Part model, mm, in its own coordinate system. Face numbers are marked on the shaded views. A direction names the side the tool comes from. Coordinates: 2 decimals unless noted, no trailing zeros. Order: outer loops, then holes, each group sorted by start corner. A loop starts at its lowest first (then second) coordinate and runs counter-clockwise, first axis right, second up.
1) Cut at C-C (y = -6.5). List the corners of the cut face in (x, z).
2) Cut at D-D (z = 24.5). List the corners of the cut face in (x, y) (3 decimals), and give its area (3 significant figures).
3) Pin check, flat tips, straight feed: pin 1 Ø6 at (y, z) = (-5.5, 20) entering from -X; pin 2 Ø1 at (y, z) = (1, 9) entering from -X; pin 3 Ø1 at (x, z) = (-1, 26) entering from +Y. Stop position of each tip, or through.
4) Wall check: L1, parallel to Y at x = 0, z = 7.5 (3 decimals); L2, parallel to Y at x = -2.75, z = 11.5; L3, parallel to X at y = -4.25, z = 8.5. Give the ranges that are in metal, low to high.
5) Cut at A-A (x = 0). List the corners of the cut face in (y, z) (3 decimals).
6) Cut at B-B (z = 15). List the corners of the cut face in (x, y) (3 decimals).
7) Mould opens along Y. For the marked faces 3, 4 and 5 say: +Y half, -Y half, draft (parallel to the pull), parting line (faces both ways), or undercut.
8) Tool access for the marked faces 1 and 2: list every direction of +Z, -Z, +X, -X, +Y, -Y with a clear straight run to the whole face (end or side of a thin tool).
```python
from build123d import *

# Parameters (mm, degrees)
SKETCH2_R           = 5.475
SKETCH1_R           = 5.61
SKETCH3_R           = 5.475
SKETCH2_2_R         = 5.475
SKETCH4_R           = 8.55
BOSS_EXTRUDE1_DEPTH = 0.68
SKETCH5_R           = 4.92
CUT_EXTRUDE1_DEPTH  = 16.57


with BuildPart() as part:
    # Sketch2 → Loft1 section 0
    with BuildSketch(Plane.XY.offset(2.23)):
        Circle(SKETCH2_R)
    # Sketch1 → Loft1 section 1
    with BuildSketch(Plane.XY):
        Circle(SKETCH1_R)
    loft()

    # Sketch3 → Loft2 section 0
    with BuildSketch(Plane.XY.offset(30.25)):
        Circle(SKETCH3_R)
    # Sketch2<2> → Loft2 section 1
    with BuildSketch(Plane.XY.offset(2.23)):
        Circle(SKETCH2_2_R)
    loft()

    # Sketch4 → Boss-Extrude1 (add)
    with BuildSketch(Plane(origin=(0, 0, 0), x_dir=(-1, 0, 0), z_dir=(0, 0, -1))):
        Circle(SKETCH4_R)
    extrude(amount=BOSS_EXTRUDE1_DEPTH)

    # Sketch5 → Cut-Extrude1 (cut)
    with BuildSketch(Plane(origin=(0, 0, -0.68), x_dir=(-1, 0, 0), z_dir=(0, 0, -1))):
        Circle(SKETCH5_R)
    extrude(amount=-CUT_EXTRUDE1_DEPTH, mode=Mode.SUBTRACT)


solid = part.part
```
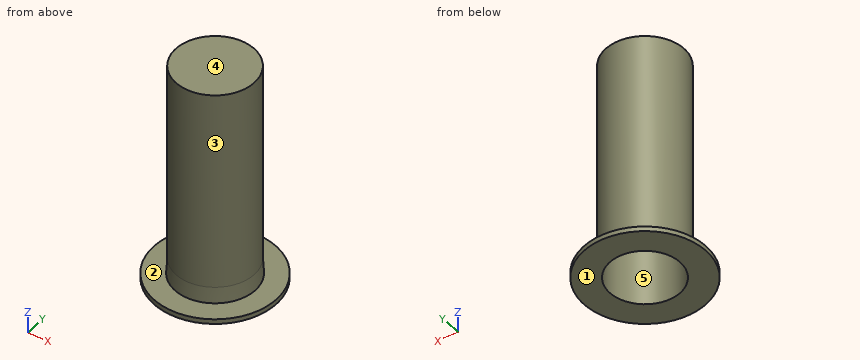
Geometry check:
1. outline: (-5.55, -0.68) - (5.55, -0.68) - (5.55, 0) - (-5.55, 0) - close
2. outline: circle Ø10.95 at (0, 0)
2. area: 94.2 mm2
3. pin 1: stops at x = -4.87
3. pin 2: stops at x = -5.45
3. pin 3: stops at y = 5.45
4. L1: y = -5.475 to -4.92, 4.92 to 5.475
4. L2: y = -4.73 to -4.08, 4.08 to 4.73
4. L3: x = -3.45 to -2.48, 2.48 to 3.45
5. outline: (-8.55, -0.68) - (-4.92, -0.68) - (-4.92, 15.89) - (4.92, 15.89) - (4.92, -0.68) - (8.55, -0.68) - (8.55, 0) - (5.61, 0) - (5.475, 2.23) - (5.475, 30.25) - (-5.475, 30.25) - (-5.475, 2.23) - (-5.61, 0) - (-8.55, 0) - close
6. outline: circle Ø10.95 at (0, 0); hole circle Ø9.84 at (0, 0)
7. face 3: parting line
7. face 4: draft
7. face 5: undercut
8. face 1: -Z, +X, -X, +Y, -Y
8. face 2: +Z
